Design review of the part built by this model. Coordinates are the model's own, in mm. Round coordinates to 2 decimals unless told otherwise and drop trailing zeros. Write each loop counter-clockwise with the first axis right and the second up, starting at its lowest first coordinate (ties: lowest second). Pieces come first, ordered by that corner, then holes.
from build123d import *

# Parameters (mm, degrees)
SKETCH1_R           = 3
SKETCH1_R_2         = 1
EXTRUDE_THIN1_DEPTH = 3
CHAMFER1_SIZE       = 0.25
CHAMFER2_SIZE       = 0.25


with BuildPart() as part:
    # Sketch1 → Extrude-Thin1 (new body)
    with BuildSketch(Plane.XY):
        Circle(SKETCH1_R)
        Circle(SKETCH1_R_2, mode=Mode.SUBTRACT)
    extrude(amount=EXTRUDE_THIN1_DEPTH)

    # Chamfer1
    chamfer1_edges = [part.edges().sort_by_distance(p)[0] for p in [
        (-3, 0, 3),
    ]]
    chamfer(chamfer1_edges, length=CHAMFER1_SIZE)

    # Chamfer2
    chamfer2_edges = [part.edges().sort_by_distance(p)[0] for p in [
        (-1, 0, 3),
    ]]
    chamfer(chamfer2_edges, length=CHAMFER2_SIZE)


solid = part.part
1) The part is to be moulded in two halves that separate along Y. For faces 1 (the face through (1, -1, 3)), 2 (the face through (-3, 0, 1)), 3 (the face through (0, -1, 1)), say which applies: pulls with the +Y half, pulls with the -Y half, needs draft (parallel to the pull), parting line crosses it, or undercut.
2) Add section A-A on y = 0. State the section outline as (x, z) points.
3) Add section C-C on z = 2.5. State the section outline as (x, y) points, and give its area (3 significant figures).
4) For line 1 along Y through (x, z) = (0, 2.1); line 2 along X through (y, z) = (-0.8, 0.85); line 3 along X through (y, z) = (0.85, 0.6), list the stretches that pass through material, from the lowest coordinate up.
Computed:
1. face 1: needs draft
1. face 2: parting line crosses it
1. face 3: undercut
2. outline: (-3, 0) - (-1, 0) - (-1, 2.75) - (-1.25, 3) - (-2.75, 3) - (-3, 2.75) - close; (1, 0) - (3, 0) - (3, 2.75) - (2.75, 3) - (1.25, 3) - (1, 2.75) - close
3. outline: circle Ø6 at (0, 0); hole circle Ø2 at (0, 0)
3. area: 25.1 mm2
4. line 1: y = -3 to -1, 1 to 3
4. line 2: x = -2.89 to -0.6, 0.6 to 2.89
4. line 3: x = -2.88 to -0.53, 0.53 to 2.88
